The model under review builds one solid part; all positions refer to its coordinate system, in mm. Give positions to 0.01 mm unless a question says otherwise; leave off trailing zeros. Order: outer loops, then holes, each group sorted by start corner. A loop starts at its lowest first (then second) coordinate and runs counter-clockwise, first axis right, second up.
```python
from build123d import *

# Parameters (mm, degrees)
SKETCH_1_R      = 28.5
SKETCH_1_R_2    = 1.6
SKETCH_1_R_3    = 15
EXTRUDE_1_DEPTH = 3
EXTRUDE_START   = -3
SKETCH_2_R      = 1.6
EXTRUDE_2_DEPTH = 3
EXTRUDE_3_DEPTH = 3


with BuildPart() as part:
    # 草图1 → 凸台-拉伸1 (new body)
    with BuildSketch(Plane.XY):
        Circle(SKETCH_1_R)
        with Locations((0, 19)):
            Circle(SKETCH_1_R_2, mode=Mode.SUBTRACT)
        Circle(SKETCH_1_R_3, mode=Mode.SUBTRACT)
        with Locations((19, 0)):
            Circle(SKETCH_1_R_2, mode=Mode.SUBTRACT)
        with Locations((0, -19)):
            Circle(SKETCH_1_R_2, mode=Mode.SUBTRACT)
        with Locations((-19, 0)):
            Circle(SKETCH_1_R_2, mode=Mode.SUBTRACT)
    extrude(amount=EXTRUDE_1_DEPTH)

    # 草图2 → 凸台-拉伸2 (add)
    with BuildSketch(Plane.XY.offset(3).offset(EXTRUDE_START)):
        with BuildLine():
            Line((24.04163056, 21.213203436), (54.800775542, -9.545941546))
            ThreePointArc((54.800775542, -9.545941546), (55.38656198, -10.960155108), (54.800775542, -12.374368671))
            Line((54.800775542, -12.374368671), (53.38656198, -13.788582233))
            ThreePointArc((53.38656198, -13.788582233), (52.817584941, -14.186984245), (52.146659903, -14.366758067))
            Line((52.146659903, -14.366758067), (35.774256751, -15.799157737))
            ThreePointArc((35.774256751, -15.799157737), (35.103331713, -15.978931559), (34.534354674, -16.377333571))
            Line((34.534354674, -16.377333571), (10.606601718, -40.305086528))
            ThreePointArc((10.606601718, -40.305086528), (9.192388155, -40.890872965), (7.778174593, -40.305086528))
            Line((7.778174593, -40.305086528), (-4.362825732, -28.164086203))
            ThreePointArc((-4.362825732, -28.164086203), (25.415604767, -12.895620742), (20.152543264, 20.152543264))
            Line((20.152543264, 20.152543264), (21.213203436, 21.213203436))
            ThreePointArc((21.213203436, 21.213203436), (22.627416998, 21.798989873), (24.04163056, 21.213203436))
        make_face()
        with Locations((50.558134855, -9.545941546)):
            Circle(SKETCH_2_R, mode=Mode.SUBTRACT)
        with Locations((36.415999231, 4.596194078)):
            Circle(SKETCH_2_R, mode=Mode.SUBTRACT)
        with Locations((17.67766953, -28.991378029)):
            Circle(SKETCH_2_R, mode=Mode.SUBTRACT)
        with Locations((31.819805153, -14.849242405)):
            Circle(SKETCH_2_R, mode=Mode.SUBTRACT)
    extrude(amount=EXTRUDE_2_DEPTH)

    # 草图4 → 凸台-拉伸3 (add)
    with BuildSketch(Plane.XY.offset(3).offset(EXTRUDE_START)):
        with BuildLine():
            Line((10.038186091, 26.673672788), (23.33185111, 21.67082656))
            ThreePointArc((23.33185111, 21.67082656), (22.205159437, 21.753906381), (21.213203436, 21.213203436))
            Line((21.213203436, 21.213203436), (20.152543264, 20.152543264))
            ThreePointArc((20.152543264, 20.152543264), (15.443487861, 23.953051636), (10.038186091, 26.673672788))
        make_face()
    extrude(amount=EXTRUDE_3_DEPTH)


solid = part.part
```
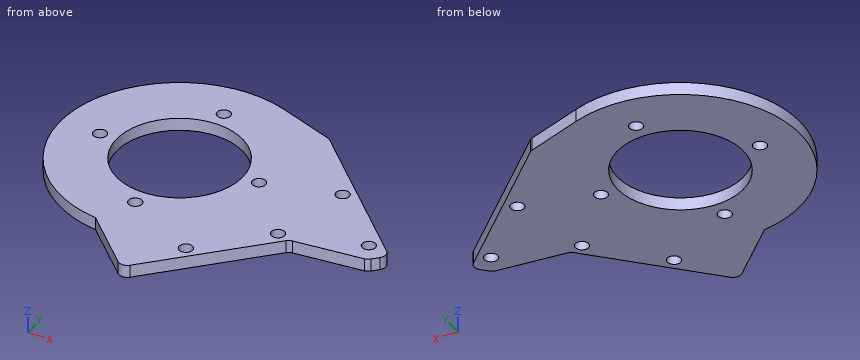
1. To check wall thickness, follow line 1 (X direction, y = 5, z = 1.25); line 2 (X direction, y = 6, z = 2.45); line 3 (Y direction, x = -2.5, z = 2.9). State the ranges of each line that lie inside material, in increasing order.
2. Insertion check: pin 1 (1.5 mm diameter, centred on y = 6, z = 1.5, fed in from -X); pin 2 (4 mm diameter, centred on x = -19, y = 0, fed in from -Z); pin 3 (3 mm diameter, centred on x = 36.42, y = 4.6, fed in from +Z). Each pin has a flat end and moves straight along its axis. Give the tip position at first contact, or say it passes through.
3. Take a section at B-B (y = 14). Write out the cut boundary in (x, z).
4. Take a section at A-A (x = -8.5). Write out the cut boundary in (y, z), and give its area (3 significant figures).
5. Take a section at C-C (z = 0.6). Count the separate pieces of the cut face and the enclosed holes in it, and give its area (3 significant figures).
6. Take a section at D-D (x = 0). Write out the cut boundary in (y, z).
Answer:
1. line 1: x = -28.06 to -14.14, 14.14 to 34.87, 37.96 to 40.25
1. line 2: x = -27.86 to -13.75, 13.75 to 35.65, 37.18 to 39.25
1. line 3: y = -30.03 to -14.79, 14.79 to 28.39
2. pin 1: stops at x = -28.01
2. pin 2: stops at z = 0
2. pin 3: passes through
3. outline: (-24.82, 0) - (-5.39, 0) - (-5.39, 3) - (-24.82, 3) - close; (5.39, 0) - (31.25, 0) - (31.25, 3) - (5.39, 3) - close
4. outline: (-27.2, 0) - (-12.36, 0) - (-12.36, 3) - (-27.2, 3) - close; (12.36, 0) - (27.2, 0) - (27.2, 3) - (12.36, 3) - close
4. area: 89.1 mm2
5. separate pieces: 1
5. enclosed holes: 9
5. area: 2,690 mm2
6. outline: (-32.53, 0) - (-20.6, 0) - (-20.6, 3) - (-32.53, 3) - close; (-17.4, 0) - (-15, 0) - (-15, 3) - (-17.4, 3) - close; (15, 0) - (17.4, 0) - (17.4, 3) - (15, 3) - close; (20.6, 0) - (28.5, 0) - (28.5, 3) - (20.6, 3) - close
